from build123d import *

# Parameters (mm, degrees)
BOSS_EXTRUDE1_DEPTH      = 10
SKETCH2_W                = 10
SKETCH2_H                = 6
BOSS_EXTRUDE2_DEPTH      = 23.975
SKETCH3_W                = 23.975
SKETCH3_H                = 6
BOSS_EXTRUDE4_DEPTH      = 2.2
BOSS_EXTRUDE4_DEPTH_BACK = 4
BOSS_EXTRUDE5_DEPTH      = 4
SKETCH5_W                = 78.65
SKETCH5_H                = 40
BOSS_EXTRUDE6_DEPTH      = 4
CUT_EXTRUDE1_DEPTH       = 79.65
FILLET1_R                = 2
SKETCH7_W                = 6
SKETCH7_H                = 6
CUT_EXTRUDE2_DEPTH       = 45
FILLET2_R                = 2
FILLET3_R                = 8
BOSS_EXTRUDE7_START      = 4
BOSS_EXTRUDE7_DEPTH      = 3
EXTRUDE_THIN1_DEPTH      = 4
FILLET4_R                = 4
FILLET5_R                = 1


with BuildPart() as part:
    # Sketch1 → Boss-Extrude1 (new body)
    with BuildSketch(Plane.XY):
        Polygon((0, 0), (-7.35, 0), (-7.35, 7.35), (-11.35, 7.35), (-11.35, -9), (4, -9), (4, 7.35), (0, 7.35), align=None)
    extrude(amount=BOSS_EXTRUDE1_DEPTH)

    # Sketch2 → Boss-Extrude2 (add)
    with BuildSketch(Plane(origin=(4, 0, 0), x_dir=(0, 0, -1), z_dir=(1, 0, 0))):
        with Locations((-5, -6)):
            Rectangle(SKETCH2_W, SKETCH2_H)
    extrude(amount=BOSS_EXTRUDE2_DEPTH)

    # Sketch3 → Boss-Extrude4 (add, two sides)
    with BuildSketch(Plane.XY.offset(10)) as boss_extrude4_sk:
        with BuildLine():
            Line((4, -2.735489451), (4, -3))
            Line((4, -3), (27.975, -3))
            Line((27.975, -3), (27.975, 5.85))
            Line((27.975, 5.85), (6.085603209, 5.85))
            ThreePointArc((6.085603209, 5.85), (6.264970626, 4.769067619), (6.325, 3.675))
            ThreePointArc((6.325, 3.675), (5.725797838, 0.265454576), (4, -2.735489451))
        make_face()
        with Locations((15.9875, -6)):
            Rectangle(SKETCH3_W, SKETCH3_H)
    extrude(amount=BOSS_EXTRUDE4_DEPTH)
    extrude(boss_extrude4_sk.sketch, amount=-BOSS_EXTRUDE4_DEPTH_BACK)

    # Sketch3<3> → Boss-Extrude5 (add)
    with BuildSketch(Plane.XY.offset(10)):
        with BuildLine():
            Line((4, 5.85), (4, -2.735489451))
            ThreePointArc((4, -2.735489451), (5.725797838, 0.265454576), (6.325, 3.675))
            ThreePointArc((6.325, 3.675), (6.264970626, 4.769067619), (6.085603209, 5.85))
            Line((6.085603209, 5.85), (4, 5.85))
        make_face()
    extrude(amount=-BOSS_EXTRUDE5_DEPTH)

    # Mirror1: part across plane


with BuildPart() as part_1:
    add(part.part)
    add(part.part.mirror(Plane.ZY.offset(-27.975)))

    # Sketch5 → Boss-Extrude6 (add)
    with BuildSketch(Plane.XY.offset(12.2)):
        with Locations((27.975, 16)):
            Rectangle(SKETCH5_W, SKETCH5_H)
    extrude(amount=BOSS_EXTRUDE6_DEPTH)

    # Sketch6 → Cut-Extrude1 (cut, through all)
    with BuildSketch(Plane(origin=(67.3, 0, 0), x_dir=(0, 0, -1), z_dir=(1, 0, 0))):
        with BuildLine():
            Line((-12.2, -9), (-10, -9))
            Line((-10, -9), (-10, -7.906246951))
            ThreePointArc((-10, -7.906246951), (-11.20325575, -6.996069572), (-12.2, -5.863484846))
            Line((-12.2, -5.863484846), (-12.2, -9))
        make_face()
        with BuildLine():
            Line((-10, -9), (-6.1, -9))
            ThreePointArc((-6.1, -9), (-8.125234291, -8.721386714), (-10, -7.906246951))
            Line((-10, -7.906246951), (-10, -9))
        make_face()
    extrude(amount=-CUT_EXTRUDE1_DEPTH, mode=Mode.SUBTRACT)

    # Fillet1
    fillet1_edges = [part_1.edges().sort_by_distance(p)[0] for p in [
        (27.975, -9, 0),
    ]]
    fillet(fillet1_edges, radius=FILLET1_R)

    # Sketch7 → Cut-Extrude2 (cut)
    with BuildSketch(Plane.XY.offset(16.2)):
        with Locations((-1.35, 26)):
            Rectangle(SKETCH7_W, SKETCH7_H)
        with Locations((13.3125, 26)):
            Rectangle(SKETCH7_W, SKETCH7_H)
        with Locations((27.975, 26)):
            Rectangle(SKETCH7_W, SKETCH7_H)
        with Locations((42.6375, 26)):
            Rectangle(SKETCH7_W, SKETCH7_H)
        with Locations((13.3125, 6)):
            Rectangle(SKETCH7_W, SKETCH7_H)
        with Locations((27.975, 6)):
            Rectangle(SKETCH7_W, SKETCH7_H)
        with Locations((42.6375, 6)):
            Rectangle(SKETCH7_W, SKETCH7_H)
        with Locations((57.3, 26)):
            Rectangle(SKETCH7_W, SKETCH7_H)
    extrude(amount=-CUT_EXTRUDE2_DEPTH, mode=Mode.SUBTRACT)

    # Fillet2
    fillet2_edges = [part_1.edges().sort_by_distance(p)[0] for p in [
        (-4.35, 23, 14.2),
        (-4.35, 29, 14.2),
        (1.65, 29, 14.2),
        (1.65, 23, 14.2),
        (54.3, 29, 14.2),
        (60.3, 29, 14.2),
        (60.3, 23, 14.2),
        (54.3, 23, 14.2),
        (45.6375, 9, 14.2),
        (45.6375, 3, 11.1),
        (39.6375, 3, 11.1),
        (39.6375, 9, 14.2),
        (30.975, 9, 14.2),
        (30.975, 3, 11.1),
        (24.975, 3, 11.1),
        (24.975, 9, 14.2),
        (10.3125, 29, 14.2),
        (16.3125, 29, 14.2),
        (16.3125, 23, 14.2),
        (10.3125, 23, 14.2),
        (24.975, 29, 14.2),
        (30.975, 29, 14.2),
        (30.975, 23, 14.2),
        (24.975, 23, 14.2),
        (39.6375, 29, 14.2),
        (45.6375, 29, 14.2),
        (45.6375, 23, 14.2),
        (39.6375, 23, 14.2),
        (16.3125, 9, 14.2),
        (16.3125, 3, 11.1),
        (10.3125, 3, 11.1),
        (10.3125, 9, 14.2),
    ]]
    fillet(fillet2_edges, radius=FILLET2_R)

    # Fillet3
    fillet3_edges = [part_1.edges().sort_by_distance(p)[0] for p in [
        (-11.35, 36, 14.2),
        (-11.35, -4, 14.2),
        (67.3, -4, 14.2),
        (67.3, 36, 14.2),
    ]]
    fillet(fillet3_edges, radius=FILLET3_R)

    # Sketch8 → Boss-Extrude7 (add)
    with BuildSketch(Plane(origin=(0, 0, 12.2), x_dir=(-1, 0, 0), z_dir=(0, 0, -1)).offset(BOSS_EXTRUDE7_START)):
        Polygon((-63.3, 32), (7.35, 32), (7.35, 19), (-7.3125, 19), (-7.3125, 0), (-48.6375, 0), (-48.6375, 19), (-63.3, 19), align=None)
    extrude(amount=BOSS_EXTRUDE7_DEPTH)

    # Sketch8<2> → Extrude-Thin1 (add)
    with BuildSketch(Plane(origin=(0, 0, 12.2), x_dir=(-1, 0, 0), z_dir=(0, 0, -1))):
        Polygon((-48.6375, 0), (-48.6375, 19), (-63.3, 19), (-63.3, 32), (7.35, 32), (7.35, 19), (-7.3125, 19), (-7.3125, 0), (-9.3125, 0), (-9.3125, 21), (5.35, 21), (5.35, 30), (-61.3, 30), (-61.3, 21), (-46.6375, 21), (-46.6375, 0), align=None)
    extrude(amount=EXTRUDE_THIN1_DEPTH)

    # Fillet4
    fillet4_edges = [part_1.edges().sort_by_distance(p)[0] for p in [
        (48.6375, 19, 8.7),
        (48.6375, 0, 5.6),
        (7.3125, 0, 5.6),
        (63.3, 32, 8.7),
        (63.3, 19, 8.7),
        (7.3125, 19, 8.7),
        (-7.35, 19, 8.7),
        (-7.35, 32, 8.7),
    ]]
    fillet(fillet4_edges, radius=FILLET4_R)

    # Fillet5
    fillet5_edges = [part_1.edges().sort_by_distance(p)[0] for p in [
        (0, 7.35, 5),
        (0, 0, 5),
        (-7.35, 0, 5),
        (-7.35, 7.35, 5),
        (55.95, 7.35, 5),
        (55.95, 0, 5),
        (63.3, 0, 5),
        (63.3, 7.35, 5),
    ]]
    fillet(fillet5_edges, radius=FILLET5_R)


solid = part_1.part
CAD build for the part. Positions are in the model's coordinates, mm. A direction names the side the tool comes from. Give positions to 0.01 mm unless a question says otherwise; leave off trailing zeros. Loops run counter-clockwise (first coordinate to the right, second up) from the corner with the lowest first, then second, coordinate; pieces in that order, holes last. Notation, with made-up numbers: M -17.5,44 L -4.5,44 A20 cw -4.5,70 Z; hole C -16.75,59 d7. An arc over 180 degrees is marked long. One line per question, with ' | ' between items. Start each with the question number.
1. Saw through at A-A on x = 33. Give the cut face in (y, z).
2. Flat gauge pins, fed straight in: pin 1 (2 mm diameter, centred on x = 27, y = 25, fed in from +Z); pin 2 (1.5 mm diameter, centred on x = 20.5, y = -5, fed in from +Z); pin 3 (2 mm diameter, centred on y = 10, z = 9.5, fed in from +X). Where does each tip first touch, or does it go through?
3. Saw through at D-D on y = 16. Give the cut face in (x, z).
4. Probe L1, parallel to Z at x = 38, y = 26; L2, parallel to Z at x = 60.5, y = -2; L3, parallel to X at y = 8, z = 10.5. List the from-to ranges inside material, lowest first. Write a range as from..to.
5. Saw through at C-C on z = 13.25. State how many separate pieces and enclosed holes the cut face has, plus the area to 3 significant figures.
6. Saw through at B-B on y = -5. Give the cut face in (x, z), plus the area to 3 significant figures.
7. Two-plate mould, pull along Y, no slides. Class faces 6 (the face through (40.21, 8.4, 14.17)), 7 (the face through (27.42, -8.4, 0.57)), 8 (the face through (25.576, 28.43, 14.172)), 9 (the face through (62.159, 30.797, 8.749)): pulls with the +Y half, pulls with the -Y half, needs draft (parallel to the pull), parting line crosses it, or undercut.
8. 3-axis set-ups, long thin cutter, end or side, ignore diameter. For faces 1 (the face through (28, 18, 12.2)), 2 (the face through (4, -5, 11)), 3 (the face through (62.097, 20.141, 8.749)), 4 (the face through (30.975, 6, 13)), 5 (the face through (0, 19, 9)): which of +Z, -Z, +X, -X, +Y, -Y reach the whole face in a straight line?
Result sheet:
1) outline: M -9,2 A2 ccw -7,0 L -3,0 L -3,6 L 0,6 L 0,5.2 L 32,5.2 L 32,12.2 L 36,12.2 L 36,16.2 L -4,16.2 L -4,12.2 L -5.86,12.2 A7.5 ccw -9,6.1 Z; hole M 5.85,8.2 L 30,8.2 L 30,12.2 L 5.85,12.2 Z
2) pin 1: stops at z = 8.2 | pin 2: stops at z = 12.2 | pin 3: stops at x = 48.64
3) outline: M -11.35,12.2 L 7.19,12.2 L 7.19,5.2 L 48.76,5.2 L 48.76,12.2 L 67.3,12.2 L 67.3,16.2 L -11.35,16.2 Z; hole M 9.31,8.2 L 46.64,8.2 L 46.64,12.2 L 9.31,12.2 Z
4) L1: z = 5.2..8.2, 12.2..16.2 | L2: z = 0..10, 12.2..16.2 | L3: x = 7.31..9.31, 46.64..48.64
5) separate pieces: 1 | enclosed holes: 8 | area: 2,830 mm^2
6) outline: M -11.35,0 L 67.3,0 L 67.3,10 L 51.95,10 L 51.95,12.2 L 4,12.2 L 4,10 L -11.35,10 Z | area: 892 mm^2
7) face 6: undercut | face 7: pulls with the -Y half | face 8: undercut | face 9: pulls with the +Y half
8) face 1: none | face 2: -X, -Y | face 3: -Z, +X | face 4: +Z | face 5: -Z, -X
